Source: three-view drawing plus pictorial views. Frame: mm from the lowest corner of the part. Give positions to 0.01 mm unless a question says otherwise; leave off trailing zeros. Loops run counter-clockwise (first coordinate to the right, second up) from the corner with the lowest first, then second, coordinate; pieces in that order, holes last. Notation, with made-up numbers: M -40,76 L 6,76 A32 cw 6,110 Z; hole C 58.25,78.5 d1. An arc over 180 degrees is marked long. Answer as a JSON object with one key per item and string values. Group by question number.
1) Ray query, L1, parallel to Z at x = 73, y = 2.3; L2, parallel to Z at x = 3, y = 1.9; L3, parallel to X at y = 1, z = 25.5. Return the intervals inside material, ascending.
2) Section query B-B on y = 1.45. Return loops of the section in (x, z), plus the area to 3 significant figures.
3) Section query C-C on x = 55.5. Return loops of the section in (y, z), plus the area to 3 significant figures.
4) Section query A-A on z = 14. Return loops of the section in (x, y), plus the area to 3 significant figures.
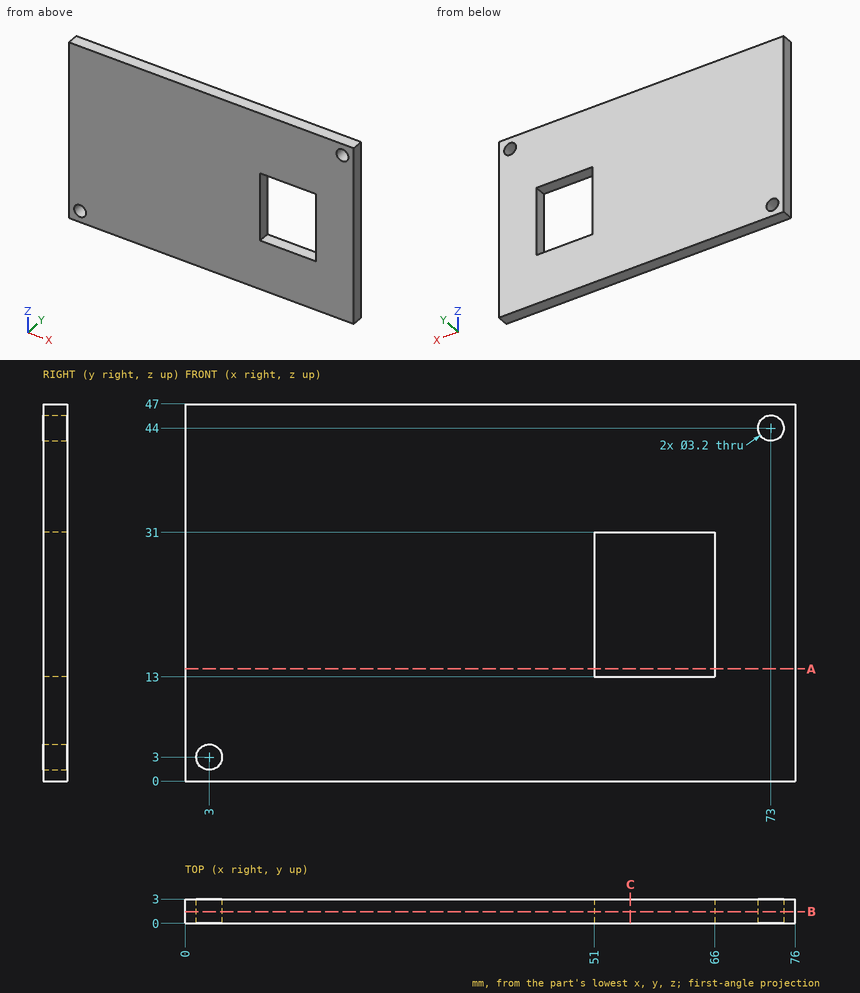
Output:
{
 "1": {"L1": "z = 0 to 42.4, 45.6 to 47", "L2": "z = 0 to 1.4, 4.6 to 47", "L3": "x = 0 to 51, 66 to 76"},
 "2": {"outline": "M 0,0 L 76,0 L 76,47 L 0,47 Z; hole C 3,3 d3.2; hole M 51,13 L 66,13 L 66,31 L 51,31 Z; hole C 73,44 d3.2", "area": "3,290 mm^2"},
 "3": {"outline": "M 0,0 L 3,0 L 3,13 L 0,13 Z; M 0,31 L 3,31 L 3,47 L 0,47 Z", "area": "87.0 mm^2"},
 "4": {"outline": "M 0,0 L 51,0 L 51,3 L 0,3 Z; M 66,0 L 76,0 L 76,3 L 66,3 Z", "area": "183 mm^2"}
}
